```python
from build123d import *

# Parameters (mm, degrees)
ESQUISSE2_R             = 8.85
ESQUISSE2_R_2           = 8
ENL_V_MAT_EXTRU_1_DEPTH = 8


with BuildPart() as part:
    # Esquisse1 → Révolution1 (revolve)
    with BuildSketch(Plane.XY, mode=Mode.PRIVATE) as r_volution1_sk:
        Polygon((2.5, 0), (13.9, 0), (13.9, 1.5), (12.4, 1.5), (12.4, 8), (13.9, 8), (13.9, 9.5), (8.85, 9.5), (8.85, 17.5), (2.5, 17.5), align=None)
    revolve(r_volution1_sk.sketch.rotate(Axis((0, 0, 0), (0, 1, 0)), 90), axis=Axis((0, 0, 0), (0, 1, 0)))

    # Esquisse2 → Enlèv. mat.-Extru.1 (cut)
    with BuildSketch(Plane(origin=(0, 17.5, 0), x_dir=(1, 0, 0), z_dir=(0, 1, 0))):
        Circle(ESQUISSE2_R)
        with Locations(Location((0, 0, 0), (0, 0, 270))):
            Circle(ESQUISSE2_R_2, mode=Mode.SUBTRACT)
    extrude(amount=-ENL_V_MAT_EXTRU_1_DEPTH, mode=Mode.SUBTRACT)


solid = part.part
```
Geometry: final body of the model. Coordinates: model frame, mm. A direction names the side the tool comes from. Round coordinates to 2 decimals unless told otherwise and drop trailing zeros. Order: outer loops, then holes, each group sorted by start corner. A loop starts at its lowest first (then second) coordinate and runs counter-clockwise, first axis right, second up. Notation, with made-up numbers: (74.25, 2) - (85.25, 2) arc R27 ccw to (85.25, 31) - close; hole circle Ø9 at (38, 63.5). An arc over 180 degrees is marked (long way). Use CSV: the item, a comma, the result in double quotes. Start each with the question number.
Q1. Mould query, pull axis Z, two halves, no side actions, for faces 1 (the face through (2, 8, -12.4)), 2 (the face through (13.57, 0.76, 3.01)), 3 (the face through (-0.1, 8.6, 2.5)). Classes: +Z half, -Z half, draft (parallel to the pull), parting line (faces both ways), or undercut.
Q2. Section query B-B (z = 0). Return loops of the section in (x, y), and give its area (3 significant figures).
Q3. Material intervals for line 1 along Y through (x, z) = (-11.25, -5.75); line 2 along X through (y, z) = (9.75, 0); line 3 along Y through (x, z) = (-7, -6.75), sorted ascending. Write a range as from..to.
Q4. First-contact query: pin 1 (5 mm diameter, centred on x = -10, y = 5, fed in from +Z); pin 2 (1.5 mm diameter, centred on x = 10, y = 3, fed in from +Z); pin 3 (1.5 mm diameter, centred on x = -9.5, z = -8, fed in from +Y); pin 4 (3 mm diameter, centred on x = 0, z = 0, fed in from +Y). Flat tips, straight axial feed; report the tip coordinate or a pass-through.
Q5. Section query D-D (x = 3). Return loops of the section in (y, z), and give its area (3 significant figures).
Q6. Section query C-C (y = 4). Return loops of the section in (x, z).
Q7. Access query for faces 4 (the face through (13.57, 8.76, 3.01)), 5 (the face through (-3.72, 4.8, -11.83)), 6 (the face through (6, 9.5, 6)). Directions: +Z, -Z, +X, -X, +Y, -Y. A direction counts if a zero-diameter tool reaches every point of the face in a straight line with its end or side. Return the directions, or none.
Q8. Section query A-A (x = 0). Return loops of the section in (y, z).
Result set:
1,face 1,"draft"
1,face 2,"parting line"
1,face 3,"undercut"
2,outline,"(-13.9, 0) - (-2.5, 0) - (-2.5, 17.5) - (-8, 17.5) - (-8, 9.5) - (-13.9, 9.5) - (-13.9, 8) - (-12.4, 8) - (-12.4, 1.5) - (-13.9, 1.5) - close; (2.5, 0) - (13.9, 0) - (13.9, 1.5) - (12.4, 1.5) - (12.4, 8) - (13.9, 8) - (13.9, 9.5) - (8, 9.5) - (8, 17.5) - (2.5, 17.5) - close"
2,area,"285 mm2"
3,line 1,"y = 0..1.5, 8..9.5"
3,line 2,"x = -8..-2.5, 2.5..8"
3,line 3,"y = 0..9.5"
4,pin 1,"stops at z = 9.87"
4,pin 2,"stops at z = 8.26"
4,pin 3,"stops at y = 9.5"
4,pin 4,"passes through"
5,outline,"(0, -13.57) - (1.5, -13.57) - (1.5, -12.03) - (8, -12.03) - (8, -13.57) - (9.5, -13.57) - (9.5, -7.42) - (17.5, -7.42) - (17.5, 7.42) - (9.5, 7.42) - (9.5, 13.57) - (8, 13.57) - (8, 12.03) - (1.5, 12.03) - (1.5, 13.57) - (0, 13.57) - close"
5,area,"357 mm2"
6,outline,"circle Ø24.8 at (0, 0); hole circle Ø5 at (0, 0)"
7,face 4,"+Y, -Y"
7,face 5,"none"
7,face 6,"+Y"
8,outline,"(0, -13.9) - (1.5, -13.9) - (1.5, -12.4) - (8, -12.4) - (8, -13.9) - (9.5, -13.9) - (9.5, -8) - (17.5, -8) - (17.5, -2.5) - (0, -2.5) - close; (0, 2.5) - (17.5, 2.5) - (17.5, 8) - (9.5, 8) - (9.5, 13.9) - (8, 13.9) - (8, 12.4) - (1.5, 12.4) - (1.5, 13.9) - (0, 13.9) - close"
